Source: three-view drawing plus pictorial views. Frame: mm from the lowest corner of the part. A direction names the side the tool comes from. Give positions to 0.01 mm unless a question says otherwise; leave off trailing zeros. Loops run counter-clockwise (first coordinate to the right, second up) from the corner with the lowest first, then second, coordinate; pieces in that order, holes last. Notation, with made-up numbers: (-33.75, -31.5) -> (-26.75, -31.5) arc R12 cw to (-26.75, -8.5) -> close; hole circle Ø4 at (-34.5, 29.25). An arc over 180 degrees is marked (long way). One line per item, written item: value. Start each with the question number.
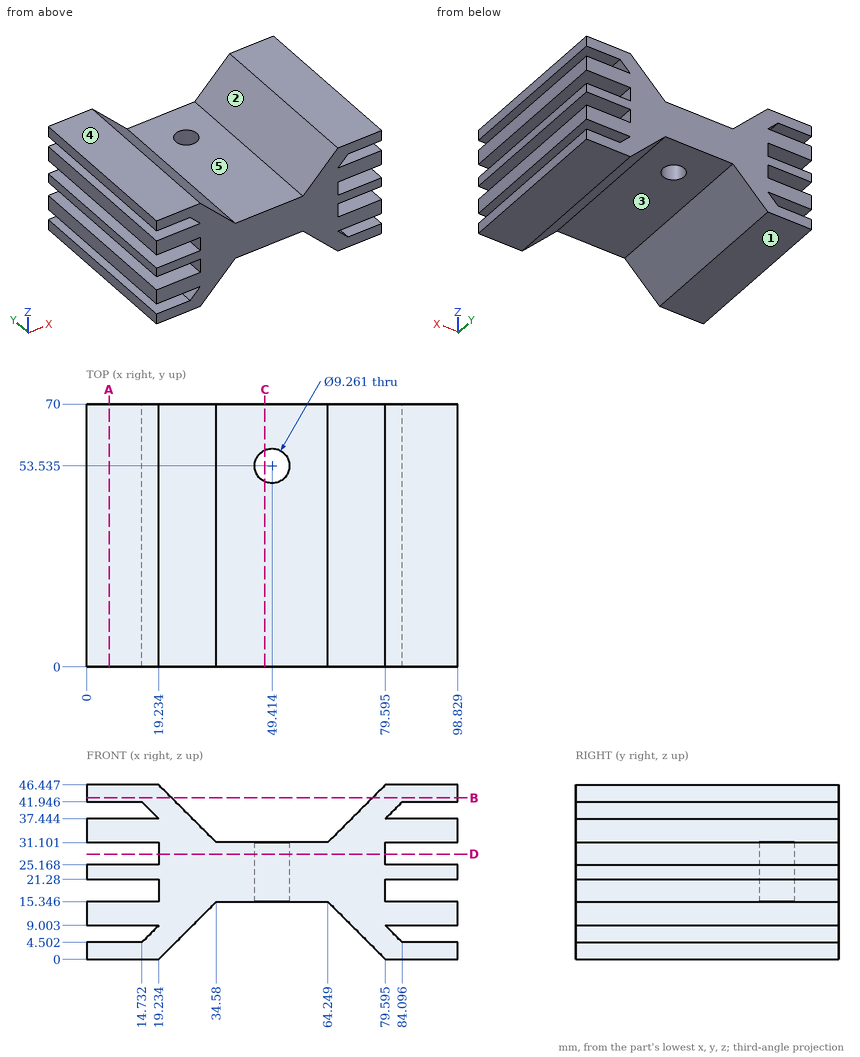
Item 1: Section D-D, the plane z = 28. Output: boundary loops of the cut face in (x, y) (1 decimal), then the cut area to 3 significant figures.
Item 2: Section A-A, the plane x = 6. Output: boundary loops of the cut face in (y, z) (1 decimal).
Item 3: Section B-B, the plane z = 43. Output: boundary loops of the cut face in (x, y).
Item 4: Section C-C, the plane x = 47.5. Output: boundary loops of the cut face in (y, z), then the cut area to 3 significant figures.
Item 5: Ray query, line 1 along Z through (x, y) = (86, 14) (1 decimal); line 2 along X through (y, z) = (54, 22); line 3 along Z through (x, y) = (47, 38). Return the intervals inside material, ascending. Write a range as [from, to].
Item 6: Pin query (flat end, axial travel): pin 1 (15 mm diameter, centred on x = 45.5, y = 50, fed in from +Z); pin 2 (4 mm diameter, centred on x = 23.5, y = 49.5, fed in from +Z); pin 3 (10 mm diameter, centred on x = 88.5, y = 61, fed in from -Z); pin 4 (2 mm diameter, centred on x = 30, y = 19.5, fed in from -Z) (1 decimal). Return the tip coordinate at first contact, or that it passes through.
Item 7: Mould query, pull axis X, two halves, no side actions, for the marked faces 4 and 5. Classes: pulls with the +X half, pulls with the -X half, needs draft (parallel to the pull), parting line crosses it, or undercut.
Item 8: Access query for the marked faces 1, 2 and 3. Directions: +Z, -Z, +X, -X, +Y, -Y. A direction counts if a zero-diameter tool reaches every point of the face in a straight line with its end or side. Return the directions, or none.
Geometry check:
1. outline: (19.2, 0) -> (79.6, 0) -> (79.6, 70) -> (19.2, 70) -> close; hole circle Ø9.3 at (49.4, 53.5)
1. area: 4,160 mm2
2. outline: (0, 0) -> (70, 0) -> (70, 4.5) -> (0, 4.5) -> close; (0, 9) -> (70, 9) -> (70, 15.3) -> (0, 15.3) -> close; (0, 21.3) -> (70, 21.3) -> (70, 25.2) -> (0, 25.2) -> close; (0, 31.1) -> (70, 31.1) -> (70, 37.4) -> (0, 37.4) -> close; (0, 41.9) -> (70, 41.9) -> (70, 46.4) -> (0, 46.4) -> close
3. outline: (0, 0) -> (22.68, 0) -> (22.68, 70) -> (0, 70) -> close; (76.15, 0) -> (98.83, 0) -> (98.83, 70) -> (76.15, 70) -> close
4. outline: (0, 15.35) -> (49.32, 15.35) -> (49.32, 31.1) -> (0, 31.1) -> close; (57.75, 15.35) -> (70, 15.35) -> (70, 31.1) -> (57.75, 31.1) -> close
4. area: 970 mm2
5. line 1: z = [0, 4.5], [9, 15.3], [21.3, 25.2], [31.1, 37.4], [41.9, 46.4]
5. line 2: x = [0, 44.81], [54.02, 98.83]
5. line 3: z = [15.35, 31.1]
6. pin 1: stops at z = 31.1
6. pin 2: stops at z = 44.18
6. pin 3: stops at z = 0
6. pin 4: stops at z = 9.8
7. face 4: needs draft
7. face 5: undercut
8. face 1: -Z, +X, -X, +Y, -Y
8. face 2: +Z, +Y, -Y
8. face 3: -Z, +Y, -Y
